```python
from build123d import *

# Parameters (mm, degrees)
SKETCH1_R           = 1
BOSS_EXTRUDE1_DEPTH = 2


with BuildPart() as part:
    # Sketch1 → Boss-Extrude1 (new body)
    with BuildSketch(Plane.XY):
        with BuildLine():
            Line((22.5, 27.5), (-22.5, 27.5))
            ThreePointArc((-22.5, 27.5), (-26.035533906, 26.035533906), (-27.5, 22.5))
            Line((-27.5, 22.5), (-27.5, -22.5))
            ThreePointArc((-27.5, -22.5), (-26.035533906, -26.035533906), (-22.5, -27.5))
            Line((-22.5, -27.5), (22.5, -27.5))
            ThreePointArc((22.5, -27.5), (26.035533906, -26.035533906), (27.5, -22.5))
            Line((27.5, -22.5), (27.5, 22.5))
            ThreePointArc((27.5, 22.5), (26.035533906, 26.035533906), (22.5, 27.5))
        make_face()
        with Locations((-22.5, 22.5)):
            Circle(SKETCH1_R, mode=Mode.SUBTRACT)
        with Locations((22.5, 22.5)):
            Circle(SKETCH1_R, mode=Mode.SUBTRACT)
        with Locations((22.5, -22.5)):
            Circle(SKETCH1_R, mode=Mode.SUBTRACT)
        with Locations((-22.5, -22.5)):
            Circle(SKETCH1_R, mode=Mode.SUBTRACT)
        with BuildLine():
            Line((-13.636038969, 22.5), (13.636038969, 22.5))
            ThreePointArc((13.636038969, 22.5), (15.945737801, 20.956708581), (15.403805922, 18.232233047))
            Line((15.403805922, 18.232233047), (1.767766953, 4.596194078))
            ThreePointArc((1.767766953, 4.596194078), (0, 3.863961031), (-1.767766953, 4.596194078))
            Line((-1.767766953, 4.596194078), (-15.403805922, 18.232233047))
            ThreePointArc((-15.403805922, 18.232233047), (-15.945737801, 20.956708581), (-13.636038969, 22.5))
        make_face(mode=Mode.SUBTRACT)
        with BuildLine():
            Line((-18.232233047, 15.403805922), (-4.596194078, 1.767766953))
            ThreePointArc((-4.596194078, 1.767766953), (-3.863961031, 0), (-4.596194078, -1.767766953))
            Line((-4.596194078, -1.767766953), (-18.232233047, -15.403805922))
            ThreePointArc((-18.232233047, -15.403805922), (-20.956708581, -15.945737801), (-22.5, -13.636038969))
            Line((-22.5, -13.636038969), (-22.5, 13.636038969))
            ThreePointArc((-22.5, 13.636038969), (-20.956708581, 15.945737801), (-18.232233047, 15.403805922))
        make_face(mode=Mode.SUBTRACT)
        with BuildLine():
            Line((-15.403805922, -18.232233047), (-1.767766953, -4.596194078))
            ThreePointArc((-1.767766953, -4.596194078), (0, -3.863961031), (1.767766953, -4.596194078))
            Line((1.767766953, -4.596194078), (15.403805922, -18.232233047))
            ThreePointArc((15.403805922, -18.232233047), (15.945737801, -20.956708581), (13.636038969, -22.5))
            Line((13.636038969, -22.5), (-13.636038969, -22.5))
            ThreePointArc((-13.636038969, -22.5), (-15.945737801, -20.956708581), (-15.403805922, -18.232233047))
        make_face(mode=Mode.SUBTRACT)
        with BuildLine():
            Line((18.232233047, -15.403805922), (4.596194078, -1.767766953))
            ThreePointArc((4.596194078, -1.767766953), (3.863961031, 0), (4.596194078, 1.767766953))
            Line((4.596194078, 1.767766953), (18.232233047, 15.403805922))
            ThreePointArc((18.232233047, 15.403805922), (20.956708581, 15.945737801), (22.5, 13.636038969))
            Line((22.5, 13.636038969), (22.5, -13.636038969))
            ThreePointArc((22.5, -13.636038969), (20.956708581, -15.945737801), (18.232233047, -15.403805922))
        make_face(mode=Mode.SUBTRACT)
    extrude(amount=BOSS_EXTRUDE1_DEPTH)


solid = part.part
```
The model under review builds one solid part; all positions refer to its coordinate system, in mm. A direction names the side the tool comes from. Round coordinates to 2 decimals unless told otherwise and drop trailing zeros. Order: outer loops, then holes, each group sorted by start corner. A loop starts at its lowest first (then second) coordinate and runs counter-clockwise, first axis right, second up.
(1) For P1, Ø1.8, axis at x = 22.5, y = -22.5, coming from the -Z side, flat-tipped, find the tip position at first contact; note if it passes through.
Working result:
P1: passes through
(2) Mouldability with a two-part tool opening along X and no side actions: class faces 1 (the face through (-27.5, 0, 1)), 2 (the face through (0, 0, 2)), 3 (the face through (8.49, -11.32, 0.99)) as released by +X, released by -X, zero draft, split by the parting line, or undercut.
Working result:
face 1: released by -X
face 2: zero draft
face 3: undercut
(3) Take a section at B-B, the plane y = 8.5. State the section outline as (x, z) points.
Working result:
outline: (-27.5, 0) - (-22.5, 0) - (-22.5, 2) - (-27.5, 2) - close; (-11.33, 0) - (-5.67, 0) - (-5.67, 2) - (-11.33, 2) - close; (5.67, 0) - (11.33, 0) - (11.33, 2) - (5.67, 2) - close; (22.5, 0) - (27.5, 0) - (27.5, 2) - (22.5, 2) - close
(4) Tool access review of faces 4 (the face through (20.92, 15.96, 0.99)), 5 (the face through (26, -26.07, 0.99)): name each direction out of +Z, -Z, +X, -X, +Y, -Y from which nothing blocks a thin tool from reaching the whole face with its end or side.
Working result:
face 4: +Z, -Z
face 5: +Z, -Z, +X, -Y
(5) Wall thickness on L1, parallel to Y at x = 0, z = 0.4; L2, parallel to X at y = 4.5, z = 0.4; L3, parallel to Y at x = -13, z = 1.35: over which ranges is each line inside the solid? List them lowest first.
Working result:
L1: y = -27.5 to -22.5, -3.86 to 3.86, 22.5 to 27.5
L2: x = -27.5 to -22.5, -7.33 to -1.67, 1.67 to 7.33, 22.5 to 27.5
L3: y = -27.5 to -22.5, -15.83 to -10.17, 10.17 to 15.83, 22.5 to 27.5
(6) Take a section at A-A, the plane x = 8. State the section outline as (y, z) points, plus the area to 3 significant figures.
Working result:
outline: (-27.5, 0) - (-22.5, 0) - (-22.5, 2) - (-27.5, 2) - close; (-10.83, 0) - (-5.17, 0) - (-5.17, 2) - (-10.83, 2) - close; (5.17, 0) - (10.83, 0) - (10.83, 2) - (5.17, 2) - close; (22.5, 0) - (27.5, 0) - (27.5, 2) - (22.5, 2) - close
area: 42.6 mm2
(7) Take a section at D-D, the plane y = -19. State the section outline as (x, z) points, plus the area to 3 significant figures.
Working result:
outline: (-27.5, 0) - (-15.93, 0) - (-15.93, 2) - (-27.5, 2) - close; (15.93, 0) - (27.5, 0) - (27.5, 2) - (15.93, 2) - close
area: 46.3 mm2
(8) Take a section at C-C, the plane z = 1.25. Count the separate pieces of the cut face and the enclosed holes in it, plus the area to 3 significant figures.
Working result:
separate pieces: 1
enclosed holes: 8
area: 1,510 mm2
